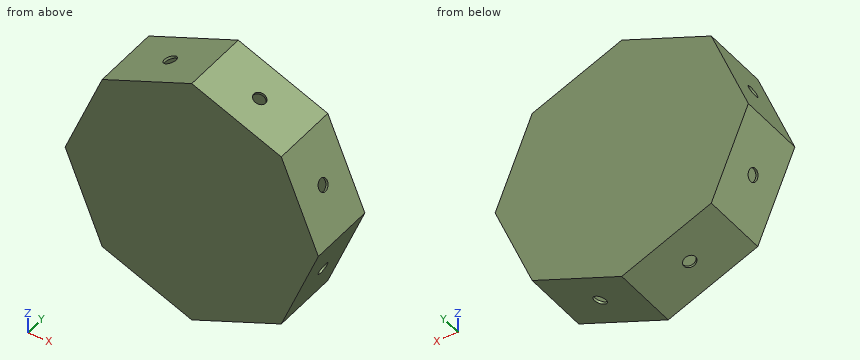
Autodesk Inventor part; units mm, degrees
ref_plane "Work Plane4" through (-100, 54, 0) normal (0, 1, 0) x (-1, 0, 0)
ref_plane "YZ Plane" through (0, 0, 0) normal (1, 0, 0) x (0, 1, 0)
ref_plane "XY Plane" through (0, 0, 0) normal (0, 0, 1) x (1, 0, 0)
sketch "Sketch1" plane through (0, 0, 0) normal (0, 1, 0) x (1, 0, 0)
  line L0 (70.7107, 70.7107) -> (-70.7107, -70.7107) construction
  line L1 (-70.7107, 70.7107) -> (70.7107, -70.7107) construction
  line L2 (-140, 0) -> (140, 0) construction
  line L3 (0, -140) -> (0, 140) construction
  line L4 (100, 0) -> (70.7107, 70.7107)
  line L5 (0, 100) -> (70.7107, 70.7107)
  line L6 (-70.7107, 70.7107) -> (0, 100)
  line L7 (-70.7107, 70.7107) -> (-100, 0)
  line L8 (-100, 0) -> (-70.7107, -70.7107)
  line L9 (-70.7107, -70.7107) -> (0, -100)
  line L10 (0, -100) -> (70.7107, -70.7107)
  line L11 (70.7107, -70.7107) -> (100, 0)
  line L12 (0, 100) -> (0, -100) construction
  line L13 (-100, 0) -> (100, 0) construction
  line L14 (98, 0) -> (69.2965, 69.2965)
  line L15 (0, 98) -> (69.2965, 69.2965)
  line L16 (0, 98) -> (-69.2965, 69.2965)
  line L17 (-69.2965, 69.2965) -> (-98, 0)
  line L18 (-98, 0) -> (-69.2965, -69.2965)
  line L19 (-69.2965, -69.2965) -> (0, -98)
  line L20 (0, -98) -> (69.2965, -69.2965)
  line L21 (69.2965, -69.2965) -> (98, 0)
  point P0 (0, 0)
  point P1 (0, 0)
  dimension "d0" = 45
  dimension "d3" = 200
  dimension "d6" = 2
extrude "Extrusion1" add sketch "Sketch1" along normal blind 54
extrude "Extrusion2" add sketch "Sketch1" along normal blind 2 contours L11 L10 L9 L8 L7 L6 L5 L4 | L21 L20 L19 L18 L17 L16 L15 L14
ref_plane "Work Plane4" through (-100, 54, 0) normal (0, 1, 0) x (-1, 0, 0)
sketch "Sketch3" plane through (-100, 54, 0) normal (0, 1, 0) x (-1, 0, 0)
  line L0 (-29.2893, -70.7107) -> (0, 0)
  line L1 (-100, -100) -> (-29.2893, -70.7107)
  line L2 (-170.7107, -70.7107) -> (-100, -100)
  line L3 (-200, 0) -> (-170.7107, -70.7107)
  line L4 (-170.7107, 70.7107) -> (-200, 0)
  line L5 (-100, 100) -> (-170.7107, 70.7107)
  line L6 (-29.2893, 70.7107) -> (-100, 100)
  line L7 (0, 0) -> (-29.2893, 70.7107)
  point P0 (-100, 0)
extrude "Extrusion4" add sketch "Sketch3" against normal blind 2
sketch "Sketch4" plane through (0, 0, 100) normal (0.3826834, 0, 0.9238795) x (0.9238795, 0, -0.3826834)
  line L0 (76.5367, 54) -> (0, 54)
  line L1 (38.2683, 54) -> (38.2683, 0) construction
  line L2 (76.5367, 0) -> (0, 0)
  line L3 (75.7713, 2) -> (0.7654, 2) construction
  point P0 (38.2683, 27)
  dimension "d15" = 25
hole "Hole1" at (35.3553, 27, 85.3553) direction (-0.3826834, 0, -0.9238795) diameter 10 depth 1.8478
pattern_circular "Circular Pattern1" count 8 over 360 about axis through (0, -10, 0) along (0, 1, 0) of "Hole1"
equation "\"d3\" = diameter"
equation "\"d6\" = thickness"
equation "\"d7\" = outher_heigth"
equation "\"d9\" = thickness"
equation "\"d13\" = thickness"
equation "\"d16\" = hole_diameter"
equation "\"diameter\" = 200"
equation "\"inner_diameter\" = diameter - 2 * thickness"
equation "\"thickness\" = 2"
equation "\"inner_heigth\" = 50"
equation "\"outher_heigth\" = inner_heigth + 2 * thickness"
equation "\"hole_pos_y\" = 0.5 * inner_heigth"
properties part number "board_case" material "PVC, Unplasticized"
Here's how the part is built. I have some questions about the finished solid (model axes, mm). Round coordinates to 2 decimals unless told otherwise and drop trailing zeros. Order: outer loops, then holes, each group sorted by start corner. A loop starts at its lowest first (then second) coordinate and runs counter-clockwise, first axis right, second up. Notation, with made-up numbers: M 42.5,47 L 52.5,47 A27 cw 52.5,66 Z; hole C 13.25,-26.75 d9. An arc over 180 degrees is marked long. Use CSV: the item, a comma, the result in double quotes.
1) I want a section at C-C (x = 5). List the corners of the cut face in (y, z) for me.
Taken from the geometry:
outline,"M 0,-97.93 L 54,-97.93 L 54,97.93 L 0,97.93 Z; hole M 2,-95.93 L 52,-95.93 L 52,95.93 L 2,95.93 Z"
2) I need wall thicknesses on line 1 along Y through (x, z) = (56, -16); line 2 along Z through (x, y) = (-14, 32); line 3 along X through (y, z) = (22, -78). Which ranges of each line are inside material? Lowest first, please. Write a range as [from, to].
Taken from the geometry:
line 1,"[0, 2], [52, 54]"
line 2,"[-94.2, -92.2], [92.2, 94.2]"
line 3,"[-53.11, -48.28], [48.28, 53.11]"
3) I want a section at A-A (y = 37.5). List the corners of the cut face in (x, z) for me, then the cut area to 3 significant figures.
Taken from the geometry:
outline,"M -100,0 L -70.71,-70.71 L 0,-100 L 70.71,-70.71 L 100,0 L 70.71,70.71 L 0,100 L -70.71,70.71 Z; hole M -98,0 L -69.3,-69.3 L 0,-98 L 69.3,-69.3 L 98,0 L 69.3,69.3 L 0,98 L -69.3,69.3 Z"
area,"1,120 mm^2"
4) I'm going to push flat-ended pins straight in: P1, Ø1, axis at y = 38.5, z = -57.5, coming from the +X side; P2, Ø12, axis at x = 57.5, y = 28, coming from the +Z side; P3, Ø1, axis at x = -42.5, y = 25, coming from the +Z side. Where does each tip first touch, or does it pass through?
Taken from the geometry:
P1,"x = 76.39"
P2,"z = 78.67"
P3,"z = 82.6"
5) I want a section at B-B (z = 21.5). List the corners of the cut face in (x, y) for me.
Taken from the geometry:
outline,"M -91.09,0 L 91.09,0 L 91.09,54 L -91.09,54 Z; hole M -89.09,2 L 89.09,2 L 89.09,52 L -89.09,52 Z"
